from build123d import *
from build123d import SkipClean  # not in build123d's __all__

# Parameters (mm, degrees)
F0_R     = 37.5
F1_DEPTH = 7
F2_R     = 6.35
F3_DEPTH = 7.001
F5_DEPTH = 7.001
F7_DEPTH = 7
F9_DEPTH = 7.001


with BuildPart() as f1:
    # F0 (on Front) → F1 (new body)
    with BuildSketch(Plane.XZ):
        Circle(F0_R)
    extrude(amount=F1_DEPTH)

    # F2 (on face) → F3 (cut, through all)
    with BuildSketch(Plane.XZ.offset(7)):
        Circle(F2_R)
    extrude(amount=-F3_DEPTH, mode=Mode.SUBTRACT)

    # F4 (on face) → F5 (cut, through all)
    with BuildSketch(Plane.XZ.offset(7)):
        with BuildLine():
            Line((-8.1433982822, 29.3566017178), (0, 37.5))
            ThreePointArc((0, 37.5), (-8.5491327229, 36.5124955281), (-16.6480090834, 33.6019909166))
            ThreePointArc((-16.6480090834, 33.6019909166), (-12.0505288232, 32.1707706914), (-8.1433982822, 29.3566017178))
        make_face()
        with BuildLine():
            ThreePointArc((16.6480090834, 33.6019909166), (8.5491327229, 36.5124955281), (0, 37.5))
            Line((0, 37.5), (8.1433982822, 29.3566017178))
            ThreePointArc((8.1433982822, 29.3566017178), (12.0505288232, 32.1707706914), (16.6480090834, 33.6019909166))
        make_face()
        with BuildLine():
            Line((0, 18.75), (0, 37.5))
            Line((0, 37.5), (-8.1433982822, 29.3566017178))
            ThreePointArc((-8.1433982822, 29.3566017178), (-4.8918070123, 24.4902514855), (-3.75, 18.75))
            Line((-3.75, 18.75), (0, 18.75))
        make_face()
        with BuildLine():
            Line((8.1433982822, 29.3566017178), (0, 37.5))
            Line((0, 37.5), (0, 18.75))
            Line((0, 18.75), (3.75, 18.75))
            ThreePointArc((3.75, 18.75), (4.8918070123, 24.4902514855), (8.1433982822, 29.3566017178))
        make_face()
        Polygon((0, 15), (0, 18.75), (-3.75, 18.75), align=None)
        Polygon((0, 15), (-3.75, 18.75), (-0.4017027864, 14.5982972136), align=None)
        Polygon((3.75, 18.75), (0, 18.75), (0, 15), align=None)
        Polygon((0.4017027864, 14.5982972136), (3.75, 18.75), (0, 15), align=None)
        with BuildLine():
            Line((-29.3566017178, -8.1433982822), (-37.5, 0))
            ThreePointArc((-37.5, 0), (-36.5124955281, -8.5491327229), (-33.6019909166, -16.6480090834))
            ThreePointArc((-33.6019909166, -16.6480090834), (-32.1707706914, -12.0505288232), (-29.3566017178, -8.1433982822))
        make_face()
        with BuildLine():
            ThreePointArc((-29.3566017178, 8.1433982822), (-32.1707706914, 12.0505288232), (-33.6019909166, 16.6480090834))
            ThreePointArc((-33.6019909166, 16.6480090834), (-36.5124955281, 8.5491327229), (-37.5, 0))
            Line((-37.5, 0), (-29.3566017178, 8.1433982822))
        make_face()
        with BuildLine():
            ThreePointArc((-18.75, 3.75), (-24.4902514855, 4.8918070123), (-29.3566017178, 8.1433982822))
            Line((-29.3566017178, 8.1433982822), (-37.5, 0))
            Line((-37.5, 0), (-18.75, 0))
            Line((-18.75, 0), (-18.75, 3.75))
        make_face()
        with BuildLine():
            Line((-18.75, 0), (-37.5, 0))
            Line((-37.5, 0), (-29.3566017178, -8.1433982822))
            ThreePointArc((-29.3566017178, -8.1433982822), (-24.4902514855, -4.8918070123), (-18.75, -3.75))
            Line((-18.75, -3.75), (-18.75, 0))
        make_face()
        Polygon((0.4017027864, 14.5982972136), (0, 15), (0, 14.1002080444), align=None)
        Polygon((0, 14.1002080444), (0, 15), (-0.4017027864, 14.5982972136), align=None)
        Polygon((-15, 0), (-18.75, 3.75), (-18.75, 0), align=None)
        Polygon((-14.5982972136, 0.4017027864), (-18.75, 3.75), (-15, 0), align=None)
        Polygon((-14.5982972136, 0.4017027864), (-15, 0), (-14.1002080444, 0), align=None)
        Polygon((-14.1002080444, 0), (-15, 0), (-14.5982972136, -0.4017027864), align=None)
        Polygon((-14.5982972136, -0.4017027864), (-15, 0), (-18.75, -3.75), align=None)
        Polygon((-15, 0), (-18.75, 0), (-18.75, -3.75), align=None)
        with BuildLine():
            ThreePointArc((-8.1433982822, -29.3566017178), (-12.0505288232, -32.1707706914), (-16.6480090834, -33.6019909166))
            ThreePointArc((-16.6480090834, -33.6019909166), (-8.5491327229, -36.5124955281), (0, -37.5))
            Line((0, -37.5), (-8.1433982822, -29.3566017178))
        make_face()
        with BuildLine():
            ThreePointArc((0, -37.5), (8.5491327229, -36.5124955281), (16.6480090834, -33.6019909166))
            ThreePointArc((16.6480090834, -33.6019909166), (12.0505288232, -32.1707706914), (8.1433982822, -29.3566017178))
            Line((8.1433982822, -29.3566017178), (0, -37.5))
        make_face()
        with BuildLine():
            Line((0, -37.5), (8.1433982822, -29.3566017178))
            ThreePointArc((8.1433982822, -29.3566017178), (4.8918070123, -24.4902514855), (3.75, -18.75))
            Line((3.75, -18.75), (0, -18.75))
            Line((0, -18.75), (0, -37.5))
        make_face()
        with BuildLine():
            Line((-8.1433982822, -29.3566017178), (0, -37.5))
            Line((0, -37.5), (0, -18.75))
            Line((0, -18.75), (-3.75, -18.75))
            ThreePointArc((-3.75, -18.75), (-4.8918070123, -24.4902514855), (-8.1433982822, -29.3566017178))
        make_face()
        Polygon((-0.4017027864, -14.5982972136), (0, -15), (0, -14.1002080444), align=None)
        Polygon((0, -14.1002080444), (0, -15), (0.4017027864, -14.5982972136), align=None)
        Polygon((0, -15), (3.75, -18.75), (0.4017027864, -14.5982972136), align=None)
        Polygon((-0.4017027864, -14.5982972136), (-3.75, -18.75), (0, -15), align=None)
        Polygon((0, -15), (-3.75, -18.75), (0, -18.75), align=None)
        Polygon((0, -18.75), (3.75, -18.75), (0, -15), align=None)
        with BuildLine():
            ThreePointArc((37.5, 0), (36.5124955281, 8.5491327229), (33.6019909166, 16.6480090834))
            ThreePointArc((33.6019909166, 16.6480090834), (32.1707706914, 12.0505288232), (29.3566017178, 8.1433982822))
            Line((29.3566017178, 8.1433982822), (37.5, 0))
        make_face()
        with BuildLine():
            Line((37.5, 0), (29.3566017178, 8.1433982822))
            ThreePointArc((29.3566017178, 8.1433982822), (24.4902514855, 4.8918070123), (18.75, 3.75))
            Line((18.75, 3.75), (18.75, 0))
            Line((18.75, 0), (37.5, 0))
        make_face()
        with BuildLine():
            ThreePointArc((33.6019909166, -16.6480090834), (36.5124955281, -8.5491327229), (37.5, 0))
            Line((37.5, 0), (29.3566017178, -8.1433982822))
            ThreePointArc((29.3566017178, -8.1433982822), (32.1707706914, -12.0505288232), (33.6019909166, -16.6480090834))
        make_face()
        with BuildLine():
            Line((29.3566017178, -8.1433982822), (37.5, 0))
            Line((37.5, 0), (18.75, 0))
            Line((18.75, 0), (18.75, -3.75))
            ThreePointArc((18.75, -3.75), (24.4902514855, -4.8918070123), (29.3566017178, -8.1433982822))
        make_face()
        Polygon((15, 0), (18.75, 3.75), (14.5982972136, 0.4017027864), align=None)
        Polygon((18.75, 0), (18.75, 3.75), (15, 0), align=None)
        Polygon((18.75, -3.75), (18.75, 0), (15, 0), align=None)
        Polygon((18.75, -3.75), (15, 0), (14.5982972136, -0.4017027864), align=None)
        Polygon((14.5982972136, -0.4017027864), (15, 0), (14.1002080444, 0), align=None)
        Polygon((14.1002080444, 0), (15, 0), (14.5982972136, 0.4017027864), align=None)
    extrude(amount=-F5_DEPTH, mode=Mode.SUBTRACT)

    # F6 (on face) → F7 (join)
    with BuildSketch(Plane.XZ.offset(7)):
        with BuildLine():
            ThreePointArc((-33.6019909166, 16.6480090834), (-26.5165042945, 26.5165042945), (-16.6480090834, 33.6019909166))
            ThreePointArc((-16.6480090834, 33.6019909166), (-29.3566017178, 29.3566017178), (-33.6019909166, 16.6480090834))
        make_face()
        with BuildLine():
            ThreePointArc((-16.6480090834, -33.6019909166), (-26.5165042945, -26.5165042945), (-33.6019909166, -16.6480090834))
            ThreePointArc((-33.6019909166, -16.6480090834), (-29.3566017178, -29.3566017178), (-16.6480090834, -33.6019909166))
        make_face()
        with BuildLine():
            ThreePointArc((33.75, -18.75), (33.7129519773, -17.6964022943), (33.6019909166, -16.6480090834))
            ThreePointArc((33.6019909166, -16.6480090834), (26.5165042945, -26.5165042945), (16.6480090834, -33.6019909166))
            ThreePointArc((16.6480090834, -33.6019909166), (28.5853987273, -30.0754108921), (33.75, -18.75))
        make_face()
        with BuildLine():
            ThreePointArc((33.75, 18.75), (28.5853987273, 30.0754108921), (16.6480090834, 33.6019909166))
            ThreePointArc((16.6480090834, 33.6019909166), (26.5165042945, 26.5165042945), (33.6019909166, 16.6480090834))
            ThreePointArc((33.6019909166, 16.6480090834), (33.7129519773, 17.6964022943), (33.75, 18.75))
        make_face()
    with SkipClean():  # cleaning this boolean's faces spoils the solid; the shape is the same uncleaned
        extrude(amount=-F7_DEPTH)

    # F8 (on face) → F9 (cut, through all)
    with BuildSketch(Plane.XZ.offset(7)):
        with BuildLine():
            ThreePointArc((-27.0181551222, 26.0051782112), (-26.5165042945, 26.5165042945), (-26.0051782112, 27.0181551222))
            ThreePointArc((-26.0051782112, 27.0181551222), (-26.5281745931, 26.5281745931), (-27.0181551222, 26.0051782112))
        make_face()
        with BuildLine():
            ThreePointArc((-27.0181551222, 26.0051782112), (-22.6262284283, 8.4555911694), (-7.75, 18.75))
            ThreePointArc((-7.75, 18.75), (-14.2116611146, 28.7701536995), (-26.0051782112, 27.0181551222))
            ThreePointArc((-26.0051782112, 27.0181551222), (-26.5165042945, 26.5165042945), (-27.0181551222, 26.0051782112))
        make_face()
        with BuildLine():
            ThreePointArc((27.0181551222, 26.0051782112), (26.5281745931, 26.5281745931), (26.0051782112, 27.0181551222))
            ThreePointArc((26.0051782112, 27.0181551222), (26.5165042945, 26.5165042945), (27.0181551222, 26.0051782112))
        make_face()
        with BuildLine():
            ThreePointArc((27.0181551222, 26.0051782112), (26.5165042945, 26.5165042945), (26.0051782112, 27.0181551222))
            ThreePointArc((26.0051782112, 27.0181551222), (8.7298463005, 14.2116611146), (29.75, 18.75))
            ThreePointArc((29.75, 18.75), (29.0444088306, 22.6262284283), (27.0181551222, 26.0051782112))
        make_face()
        with BuildLine():
            ThreePointArc((26.0051782112, -27.0181551222), (26.5281745931, -26.5281745931), (27.0181551222, -26.0051782112))
            ThreePointArc((27.0181551222, -26.0051782112), (26.5165042945, -26.5165042945), (26.0051782112, -27.0181551222))
        make_face()
        with BuildLine():
            ThreePointArc((26.0051782112, -27.0181551222), (26.5165042945, -26.5165042945), (27.0181551222, -26.0051782112))
            ThreePointArc((27.0181551222, -26.0051782112), (29.0444088306, -22.6262284283), (29.75, -18.75))
            ThreePointArc((29.75, -18.75), (8.7298463005, -14.2116611146), (26.0051782112, -27.0181551222))
        make_face()
        with BuildLine():
            ThreePointArc((-26.0051782112, -27.0181551222), (-26.5165042945, -26.5165042945), (-27.0181551222, -26.0051782112))
            ThreePointArc((-27.0181551222, -26.0051782112), (-26.5281745931, -26.5281745931), (-26.0051782112, -27.0181551222))
        make_face()
        with BuildLine():
            ThreePointArc((-7.75, -18.75), (-22.6262284283, -8.4555911694), (-27.0181551222, -26.0051782112))
            ThreePointArc((-27.0181551222, -26.0051782112), (-26.5165042945, -26.5165042945), (-26.0051782112, -27.0181551222))
            ThreePointArc((-26.0051782112, -27.0181551222), (-14.2116611146, -28.7701536995), (-7.75, -18.75))
        make_face()
    extrude(amount=-F9_DEPTH, mode=Mode.SUBTRACT)


solid = f1.part
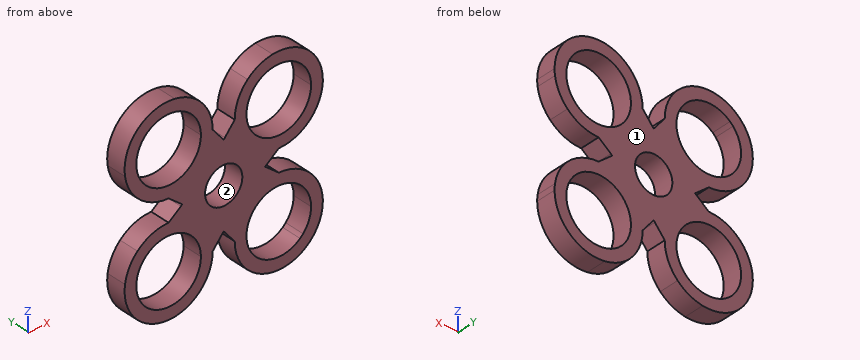
The listing builds one solid part. Answer for the finished solid, in the listing's coordinates (mm). Face numbers are marked on the shaded views. Coordinates: 2 decimals unless noted, no trailing zeros. Write each loop counter-clockwise with the first axis right and the second up, starting at its lowest first coordinate (ties: lowest second). Pieces come first, ordered by that corner, then holes. Notation, with made-up numbers: M 2.25,-12.75 L 61.25,-12.75 A29 cw 61.25,16.25 Z; hole C 17.25,-35.5 d4. An arc over 180 degrees is marked long. Put each result on its own line as item: value. Start each with the question number.
1. Consider line 1 (Z direction, x = 18.75, y = -4). Determine where the line is inside the solid, lowest interval first. Write a range as from..to.
2. For a pull along X with two mould halves and no side action, classify the marked faces 1 and 2 as pulls with the +X half, pulls with the -X half, needs draft (parallel to the pull), parting line crosses it, or undercut.
3. A cutting plane is placed at B-B on y = -5.5. Write down the section's boundary in (x, z), then the cut area to 3 significant figures.
4. A cutting plane is placed at A-A on x = -21. Write down the section's boundary in (y, z).
5. Flat-ended cylindrical pins translate along their axes: P1, Ø1, axis at x = 24, y = -6, coming from the +Z side; P2, Ø13, axis at x = -18.75, z = 18.75, coming from the -Y side; P3, Ø3, axis at x = -13.5, y = -3, coming from the +Z side. Find the tip coordinate at first contact, or state that the pin passes through.
6. A cutting plane is placed at C-C on x = 28.5. Write down the section's boundary in (y, z), then the cut area to 3 significant figures.
Resolved:
1. line 1: z = -33.75..-29.75, -7.75..-3.75, 3.75..7.75, 29.75..33.75
2. face 1: needs draft
2. face 2: undercut
3. outline: M -18.75,-3.75 A15 ccw long -3.75,-18.75 L 0,-14.1 L 3.75,-18.75 A15 ccw long 18.75,-3.75 L 14.1,0 L 18.75,3.75 A15 ccw long 3.75,18.75 L 0,14.1 L -3.75,18.75 A15 ccw long -18.75,3.75 L -14.1,0 Z; hole C -18.75,-18.75 d22; hole C -18.75,18.75 d22; hole C 0,0 d12.7; hole C 18.75,-18.75 d22; hole C 18.75,18.75 d22
3. area: 1,810 mm2
4. outline: M -7,-33.58 L 0,-33.58 L 0,-29.52 L -7,-29.52 Z; M -7,-7.98 L 0,-7.98 L 0,-3.92 L -7,-3.92 Z; M -7,3.92 L 0,3.92 L 0,7.98 L -7,7.98 Z; M -7,29.52 L 0,29.52 L 0,33.58 L -7,33.58 Z
5. P1: stops at z = 32.98
5. P2: passes through
5. P3: stops at z = 33.27
6. outline: M -7,-30.15 L 0,-30.15 L 0,-23.84 L -7,-23.84 Z; M -7,-13.66 L 0,-13.66 L 0,-7.35 L -7,-7.35 Z; M -7,7.35 L 0,7.35 L 0,13.66 L -7,13.66 Z; M -7,23.84 L 0,23.84 L 0,30.15 L -7,30.15 Z
6. area: 177 mm2
